Input: part model. Units: mm. Frame: model coordinates. A direction names the side the tool comes from. Round coordinates to 2 decimals unless told otherwise and drop trailing zeros. Loops run counter-clockwise (first coordinate to the right, second up) from the corner with the lowest first, then second, coordinate; pieces in that order, holes last. Notation, with made-up numbers: (39, 68.5) - (46, 68.5) arc R26 cw to (46, 85.5) - close; hole circle Ø11 at (82.5, 61.5). An arc over 180 degrees is marked (long way). One line per question, with ' | ' between items. Start each with the question number.
Item 1: First-contact query: pin 1 (2.5 mm diameter, centred on x = 8.5, z = -1, fed in from -Y); pin 2 (1.6 mm diameter, centred on y = 0.5, z = -1.5, fed in from +X); pin 3 (1 mm diameter, centred on y = 2.5, z = 3.5, fed in from +X). Flat tips, straight axial feed; report the tip coordinate or a pass-through.
Item 2: Set-up query: faces 4 (the face through (6, 1, -6.7)), 5 (the face through (7, 3.2, 0)), 6 (the face through (9.872, 1.014, 2.024)). Return all of +Z, -Z, +X, -X, +Y, -Y with unobstructed straight access to the full face (end or side cutting, diameter ignored); none if empty.
Item 3: Material intervals for line 1 along X through (y, z) = (0.6, 0); line 2 along Z through (x, y) = (4.5, 1.4); line 3 along Z through (x, y) = (7.5, 0.6), sorted ascending.
Item 4: Section C-C, the plane y = 2.75. Return loops of the section in (x, z).
Item 5: Draft query along X for faces 1 (the face through (6, 2, 2)), 2 (the face through (1, 0, 1)), 3 (the face through (12.36, 2.29, -0.7)). Return one class per face: pulls with the +X half, pulls with the -X half, needs draft (parallel to the pull), parting line crosses it, or undercut.
Item 6: Section D-D, the plane z = -3.5. Return loops of the section in (x, y), plus the area to 3 significant figures.
Item 7: Section A-A, the plane y = 1.5. Return loops of the section in (x, z), plus the area to 3 significant figures.
Item 8: Section B-B, the plane x = 4. Return loops of the section in (y, z).
```python
from build123d import *

# Parameters (mm, degrees)
MAINBASESKETCH_W          = 15.8
MAINBASESKETCH_H          = 3.2
MAINBASEEXTRUDE_DEPTH     = 7.9
MAINBASESHELL_T           = -1.2
UNDERSIDECIRCLEEXT_START  = -0.2
UNDERSIDECIRCLESKETCH_R   = 3.05
UNDERSIDECIRCLESKETCH_R_2 = 2.4
UNDERSIDECIRCLEEXT_DEPTH  = 2.2
SECONDANGLEDCUT_DEPTH     = 19.555463972
SECONDNOTCH_DEPTH         = 2.2


with BuildPart() as part:
    # MainBaseSketch → MainBaseExtrude (new, symmetric)
    with BuildSketch(Plane.XY):
        with Locations((8.581967213, 1.6)):
            Rectangle(MAINBASESKETCH_W, MAINBASESKETCH_H)
    extrude(amount=MAINBASEEXTRUDE_DEPTH, both=True)

    # MainBaseShell
    mainbaseshell_openings = [part.faces().sort_by_distance(p)[0] for p in [
        (8.581967213, 0, 0),
    ]]
    offset(amount=MAINBASESHELL_T, openings=mainbaseshell_openings, kind=Kind.INTERSECTION)

    # UnderSideCircleSketch → UnderSideCircleExt (add)
    with BuildSketch(Plane.XZ.offset(-2).offset(UNDERSIDECIRCLEEXT_START)):
        with Locations((8.581967213, 0)):
            Circle(UNDERSIDECIRCLESKETCH_R)
        with Locations((8.581967213, 0)):
            Circle(UNDERSIDECIRCLESKETCH_R_2, mode=Mode.SUBTRACT)
    extrude(amount=UNDERSIDECIRCLEEXT_DEPTH)

    # Sketch53 → SecondAngledCut (cut, through all)
    with BuildSketch(Plane(origin=(0, 0, 0), x_dir=(-1, 0, 0), z_dir=(0, -1, 0))):
        Polygon((-8.833667893, 7.9), (-15.981967213, -6.7), (-15.981967213, -7.9), (-16.481967213, -7.9), (-16.481967213, 7.9), align=None)
    extrude(amount=-SECONDANGLEDCUT_DEPTH, mode=Mode.SUBTRACT)

    # Sketch56 → SecondNotch (cut)
    with BuildSketch(Plane(origin=(0, 0, 0), x_dir=(-1, 0, 0), z_dir=(0, -1, 0))):
        with BuildLine():
            Line((-10.711153505, 3.699172992), (-11.897271127, 1.358994981))
            ThreePointArc((-11.897271127, 1.358994981), (-11.034832221, 2.39254887), (-10.711153505, 3.699172992))
        make_face()
    extrude(amount=-SECONDNOTCH_DEPTH, mode=Mode.SUBTRACT)


solid = part.part
```
Return value:
1) pin 1: y = 2 | pin 2: x = 11.55 | pin 3: x = 14.66
2) face 4: +X, -Y | face 5: +Z, -Z, +X, -X, +Y | face 6: -Y
3) line 1: 0.68 to 1.88, 5.53 to 6.18, 10.98 to 11.63 | line 2: -7.9 to -6.7, 6.7 to 7.9 | line 3: -7.9 to -6.7, -2.85 to -2.14, 2.14 to 2.85, 6.7 to 7.9
4) outline: (0.68, -7.9) - (8.83, -7.9) - (15.98, 6.7) - (15.98, 7.9) - (0.68, 7.9) - close
5) face 1: undercut | face 2: needs draft | face 3: pulls with the +X half
6) outline: (0.68, 0) - (1.88, 0) - (1.88, 2) - (10.72, 2) - (10.72, 2.2) - (10.81, 2.2) - (10.81, 2) - (10.99, 2) - (10.99, 3.2) - (0.68, 3.2) - close | area: 14.7 mm2
7) outline: (0.68, -7.9) - (8.83, -7.9) - (9.42, -6.7) - (1.88, -6.7) - (1.88, 6.7) - (15.28, 6.7) - (15.28, 5.27) - (15.98, 6.7) - (15.98, 7.9) - (0.68, 7.9) - close; circle Ø6.1 at (8.58, 0); hole circle Ø4.8 at (8.58, 0) | area: 56.2 mm2
8) outline: (0, -7.9) - (3.2, -7.9) - (3.2, 7.9) - (0, 7.9) - (0, 6.7) - (2, 6.7) - (2, -6.7) - (0, -6.7) - close
